Geometry check sheet. Reference: drawing and pictorial views, mm from the part's lowest x, y, z. Give positions to 0.01 mm unless a question says otherwise; leave off trailing zeros. Write each loop counter-clockwise with the first axis right and the second up, starting at its lowest first coordinate (ties: lowest second). Pieces come first, ordered by that corner, then holes.
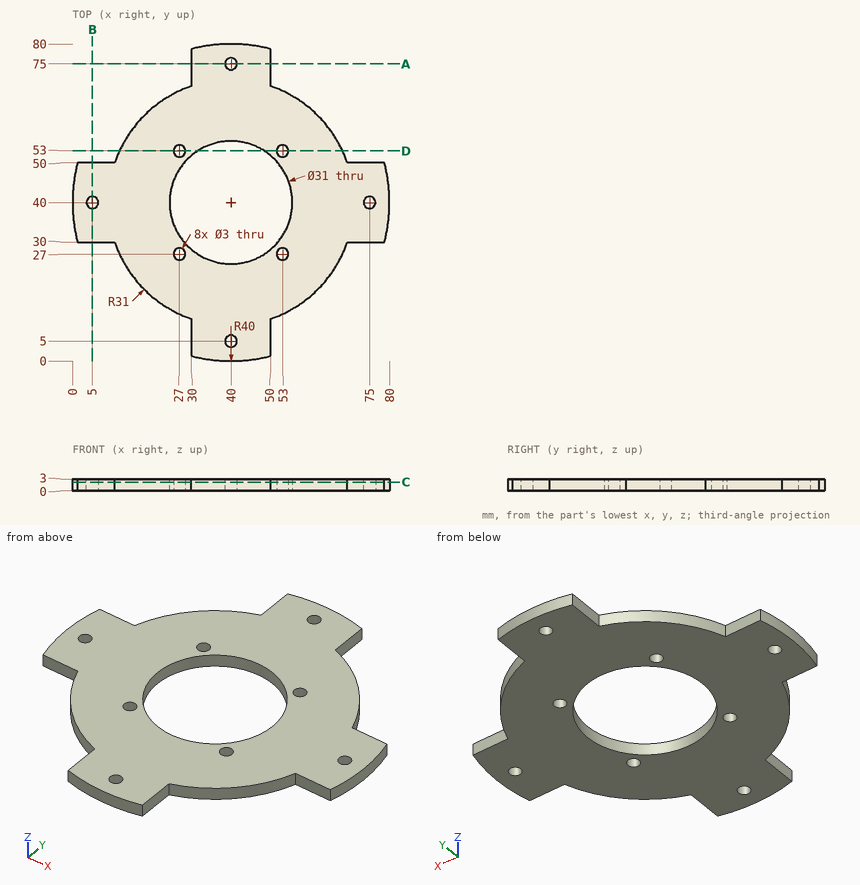
Item 1: Sectioned sample at A-A on y = 75. Record the cut outline in (x, z).
Answer key:
outline: (30, 0) - (38.5, 0) - (38.5, 3) - (30, 3) - close; (41.5, 0) - (50, 0) - (50, 3) - (41.5, 3) - close
Item 2: Sectioned sample at C-C on z = 2.2. State how many separate pieces and enclosed holes the cut face has, then the cut area to 3 significant figures.
Answer key:
separate pieces: 1
enclosed holes: 9
area: 2,940 mm2
Item 3: Depth check by flat-ended pin: pin 1 (2.5 mm diameter, centred on x = 53, y = 27, fed in from -Z); pin 2 (1 mm diameter, centred on y = 35.5, z = 1.5, fed in from -X); pin 3 (1.5 mm diameter, centred on y = 7.5, z = 2, fed in from +X); pin 4 (1.5 mm diameter, centred on y = 75, z = 1.5, fed in from -X). Enter the tip coordinate at first touch or a pass-through.
Answer key:
pin 1: passes through
pin 2: stops at x = 0.2
pin 3: stops at x = 50
pin 4: stops at x = 30
Item 4: Scan lines: line 1 along Y through (x, z) = (40, 2.3); line 2 along X through (y, z) = (54, 0.4); line 3 along Y through (x, z) = (53, 1.5). Record each from-to range of solid material in increasing order.
Answer key:
line 1: y = 0 to 3.5, 6.5 to 24.5, 55.5 to 73.5, 76.5 to 80
line 2: x = 12.34 to 25.88, 28.12 to 33.35, 46.65 to 51.88, 54.12 to 67.66
line 3: y = 11.86 to 25.5, 28.5 to 31.56, 48.44 to 51.5, 54.5 to 68.14
Item 5: Sectioned sample at D-D on y = 53. Record the cut outline in (x, z).
Answer key:
outline: (11.86, 0) - (25.5, 0) - (25.5, 3) - (11.86, 3) - close; (28.5, 0) - (31.56, 0) - (31.56, 3) - (28.5, 3) - close; (48.44, 0) - (51.5, 0) - (51.5, 3) - (48.44, 3) - close; (54.5, 0) - (68.14, 0) - (68.14, 3) - (54.5, 3) - close
